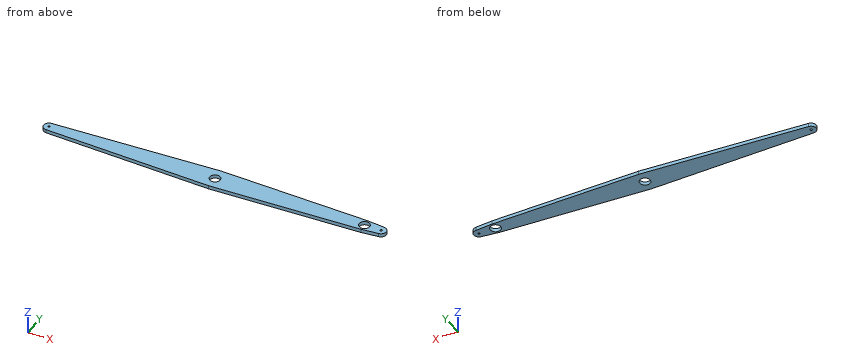
from build123d import *

# Parameters (mm, degrees)
SKIZZE1_R                       = 30
SKIZZE1_R_2                     = 6
AUFSATZ_LINEAR_AUSTRAGEN1_DEPTH = 20


with BuildPart() as part:
    # Skizze1 → Aufsatz-Linear austragen1 (new body)
    with BuildSketch(Plane.XY):
        with BuildLine():
            Line((-950, 70), (-95, 40))
            Line((-95, 40), (0, 30))
            ThreePointArc((0, 30), (30, 0), (0, -30))
            Line((0, -30), (-95, -40))
            Line((-95, -40), (-950, -70))
            Line((-950, -70), (-1900, -30))
            ThreePointArc((-1900, -30), (-1930, 0), (-1900, 30))
            Line((-1900, 30), (-950, 70))
        make_face()
        with Locations((-950, 0)):
            Circle(SKIZZE1_R, mode=Mode.SUBTRACT)
        with Locations((-95, 0)):
            Circle(SKIZZE1_R, mode=Mode.SUBTRACT)
        with Locations((-1900, 0)):
            Circle(SKIZZE1_R_2, mode=Mode.SUBTRACT)
        Circle(SKIZZE1_R_2, mode=Mode.SUBTRACT)
    extrude(amount=AUFSATZ_LINEAR_AUSTRAGEN1_DEPTH)


solid = part.part
Can you work these out from the model? Positions are in its coordinate system, mm. Round coordinates to 2 decimals unless told otherwise and drop trailing zeros. Loops run counter-clockwise (first coordinate to the right, second up) from the corner with the lowest first, then second, coordinate; pieces in that order, holes last. Notation, with made-up numbers: (52, 21) - (87, 21) arc R18 ccw to (87, 48) - close; hole circle Ø2 at (12.25, 6). An arc over 180 degrees is marked (long way). Answer in a Markdown table with one row per item. Add a question column.
Q1. I need wall thicknesses on L1, parallel to X at y = -23, z = 9.25; L2, parallel to X at y = 25, z = 9.5; L3, parallel to Y at x = -95, z = 9. Which ranges of each line are inside material? Lowest first, please.
Q2. For pin 1 Ø12 at (x, z) = (-449, 13) entering from +Y; pin 2 Ø3 at (y, z) = (-20.5, 5) entering from -X; pin 3 Ø6 at (y, z) = (5, 11) entering from -X, each with a flat end and sliding along its axis, tell me the tip position at first contact or that it passes through.
Q3. I want a section at B-B on x = -726. List the corners of the cut face in (y, z) for me.
Q4. I want a section at A-A on z = 15.75. List the corners of the cut face in (x, y) for me, and give its area (3 significant figures).
Q5. I want a section at C-C on x = -374.5. List the corners of the cut face in (y, z) for me, and give its area (3 significant figures).
A:
| question | item | result |
|---|---|---|
| 1 | L1 | -1919.26 to -969.26, -930.74 to -114.26, -75.74 to 19.26 |
| 1 | L2 | -1916.58 to -966.58, -933.42 to -111.58, -78.42 to 16.58 |
| 1 | L3 | -40 to -30, 30 to 40 |
| 2 | pin 1 | y = 52.63 |
| 2 | pin 2 | x = -1923.22 |
| 2 | pin 3 | x = -1929.93 |
| 3 | outline | (-62.14, 0) - (62.14, 0) - (62.14, 20) - (-62.14, 20) - close |
| 4 | outline | (-1900, -30) - (-950, -70) - (-95, -40) - (0, -30) arc R30 ccw to (0, 30) - (-95, 40) - (-950, 70) - (-1900, 30) arc R30 ccw to start; hole circle Ø12 at (-1900, 0); hole circle Ø60 at (-950, 0); hole circle Ø60 at (-95, 0); hole circle Ø12 at (0, 0) |
| 4 | area | 193,000 mm^2 |
| 5 | outline | (-49.81, 0) - (49.81, 0) - (49.81, 20) - (-49.81, 20) - close |
| 5 | area | 1,990 mm^2 |
